Geometry check sheet. Reference: drawing and pictorial views, mm from the part's lowest x, y, z. A direction names the side the tool comes from. Round coordinates to 2 decimals unless told otherwise and drop trailing zeros. Write each loop counter-clockwise with the first axis right and the second up, starting at its lowest first coordinate (ties: lowest second). Pieces come first, ordered by that corner, then holes. Notation, with made-up numbers: M 79.5,89.25 L 106.5,89.25 A36 cw 106.5,124.25 Z; hole C 49,46 d4. An arc over 180 degrees is marked long. Put each result on its own line as item: value. Start each with the question number.
(1) Material ranges on probe 1 along Z at (x, y) = (59, 16); probe 2 along X at (y, z) = (10.5, 16); probe 3 along X at (y, z) = (28.5, 4.25), recorded low to high.
(2) Gauge pin test, flat ends, axial feed: pin 1 (12 mm diameter, centred on y = 26, z = 14.5, fed in from -X); pin 2 (8 mm diameter, centred on x = 47, z = 8.5, fed in from -Y). Record the tip position at first contact, or that the pin passes through.
(3) Mould release check, pull along X, two halves, no side actions. Record for the marked faces 3, 4 and 5: pulls with the +X half, pulls with the -X half, needs draft (parallel to the pull), parting line crosses it, or undercut.
(4) Section check C-C on x = 48. Record the cut outline in (y, z).
(5) Tool access check on the marked faces 1 and 2. Record the directions out of +Z, -Z, +X, -X, +Y, -Y that give a thin tool (end or side, any length) a straight path to the whole face; none if there is none.
(6) Section check A-A on y = 46. Record the cut outline in (x, z).
(7) Section check D-D on z = 14.75. Record the cut outline in (x, y).
(8) Section check B-B on z = 10. Record the cut outline in (x, y).
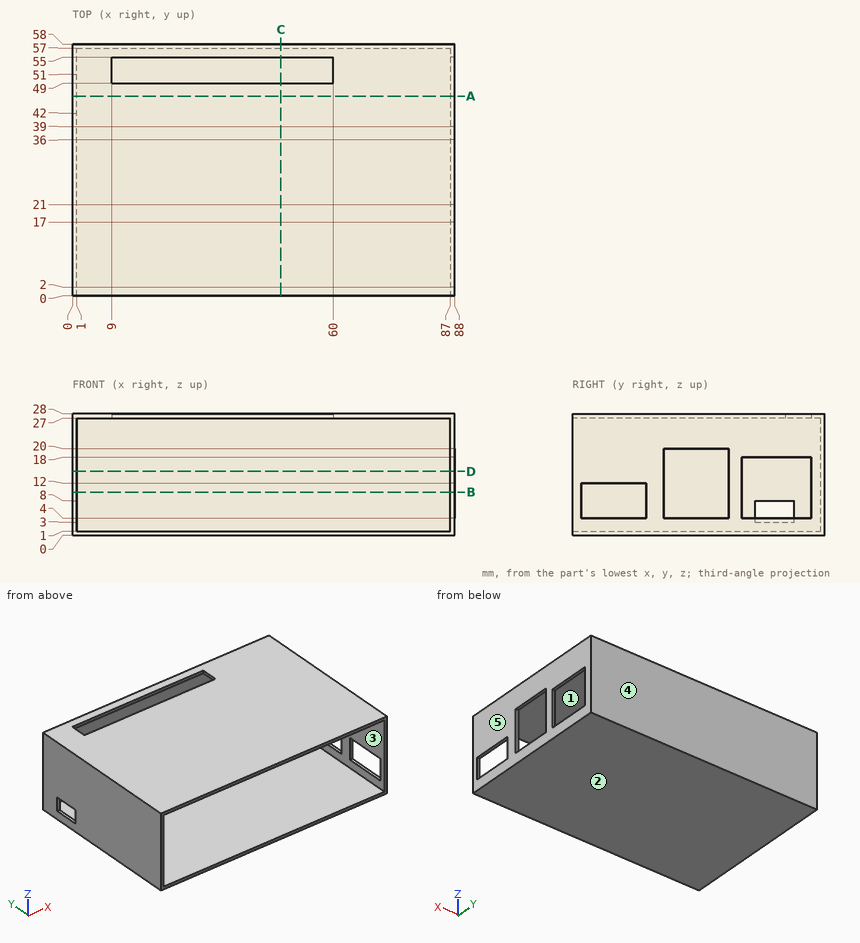
Answers follow:
1. probe 1: z = 0 to 1, 27 to 28
1. probe 2: x = 0 to 1, 87 to 88
1. probe 3: x = 0 to 1
2. pin 1: stops at x = 0
2. pin 2: stops at y = 57
3. face 3: undercut
3. face 4: needs draft
3. face 5: pulls with the +X half
4. outline: M 0,0 L 58,0 L 58,28 L 55,28 L 55,27 L 57,27 L 57,1 L 0,1 Z; M 0,27 L 49,27 L 49,28 L 0,28 Z
5. face 1: -Y
5. face 2: -Z, +X, -X, +Y, -Y
6. outline: M 0,0 L 88,0 L 88,4 L 87,4 L 87,1 L 1,1 L 1,3 L 0,3 Z; M 0,8 L 1,8 L 1,27 L 87,27 L 87,18 L 88,18 L 88,28 L 0,28 Z
7. outline: M 0,0 L 1,0 L 1,57 L 87,57 L 87,55 L 88,55 L 88,58 L 0,58 Z; M 87,0 L 88,0 L 88,21 L 87,21 Z; M 87,36 L 88,36 L 88,39 L 87,39 Z
8. outline: M 0,0 L 1,0 L 1,57 L 87,57 L 87,55 L 88,55 L 88,58 L 0,58 Z; M 87,0 L 88,0 L 88,2 L 87,2 Z; M 87,17 L 88,17 L 88,21 L 87,21 Z; M 87,36 L 88,36 L 88,39 L 87,39 Z
